Autodesk Inventor part; units mm, degrees
ref_plane "YZ Plane" through (0, 0, 0) normal (1, 0, 0) x (0, 1, 0)
ref_plane "XZ Plane" through (0, 0, 0) normal (0, 1, 0) x (-1, 0, 0)
ref_plane "XY Plane" through (0, 0, 0) normal (0, 0, 1) x (1, 0, 0)
sketch "Эскиз1" plane through (0, 0, 0) normal (0, 0, 1) x (1, 0, 0)
  line L0 (0, 0) -> (18, 0)
  line L1 (18, 0) -> (18, 18)
  line L2 (18, 18) -> (0, 18)
  line L3 (0, 18) -> (0, 0)
  dimension "d0" = 18
  dimension "d1" = 18
extrude "Выдавливание1" add sketch "Эскиз1" along normal blind 2
sketch "Эскиз4" plane through (0, 0, 0) normal (0, 0, -1) x (-1, 0, 0)
  circle A0 centre (-9, 9) radius 4.05
  line L0 (-18, 0) -> (-18, 18)
  line L1 (-18, 9) -> (0, 9)
  line L2 (0, 18) -> (0, 0)
  dimension "d14" = 8.1
extrude "Выдавливание3" cut sketch "Эскиз4" against normal blind 0.3
sketch "Эскиз5" plane through (0, 0, 2) normal (0, 0, 1) x (1, 0, 0)
  circle A0 centre (9, 9) radius 1.75
  circle A1 centre (9, 9) radius 5.714
  line L0 (0, 18) -> (0, 0)
  line L1 (6.1362, 11.8638) -> (0, 18)
  line L2 (18, 0) -> (18, 18)
  line L3 (11.8638, 11.8638) -> (18, 18)
  line L4 (0, 0) -> (18, 0)
  line L5 (0, 0) -> (6.1362, 6.1362)
  line L6 (18, 0) -> (11.8638, 6.1362)
  circle A2 centre (9, 9) radius 4.05
  line L7 (3.0681, 14.9319) -> (4.0681, 14.9319)
  line L8 (3.0681, 3.0681) -> (4.0681, 3.0681)
  line L9 (14.9319, 3.0681) -> (13.9319, 3.0681)
  line L10 (14.9319, 14.9319) -> (13.9319, 14.9319)
  dimension "d24" = 1
hole "Отверстие2" at (4.0681, 14.9319, 2) at (4.0681, 3.0681, 2) at (13.9319, 14.9319, 2) at (13.9319, 3.0681, 2) direction (0, 0, -1) diameter 2.2 depth 5 countersink diameter 4 countersink angle 90
fillet "Сопряжение1" radius 1.05 2 edges at (9, 0, 2) (9, 18, 2)
fillet "Сопряжение1" radius 2.05 2 edges at (18, 9, 2) (0, 9, 2)
sketch "Эскиз6" plane through (9, 9, 0.3) normal (0, 0, -1) x (-1, 0, 0)
  circle A0 centre (0, 0) radius 1.75
  point P0 (9, -9)
  dimension "d27" = 3.5
extrude "Выдавливание4" cut sketch "Эскиз6" against normal through all
properties part number "Крышка поворотного кулака"
Could you check a few things on this model? Use its own coordinates, in mm. A direction names the side the tool comes from. Round coordinates to 2 decimals unless told otherwise and drop trailing zeros. Write each loop counter-clockwise with the first axis right and the second up, starting at its lowest first coordinate (ties: lowest second). Pieces come first, ordered by that corner, then holes. Notation, with made-up numbers: M -14,41.25 L 38,41.25 A20 ccw 38,69.25 Z; hole C -1,35.5 d1. An arc over 180 degrees is marked long. Answer in a Markdown table with one row per item. Add a question column.
Q1. Imagine slicing it at B-B (y = 9). Please give me the cut outline in (x, z), then the cut area to 3 significant figures.
Q2. Will these pins go through, and if not, where does the flat tip stop? pin 1 Ø3 at (x, y) = (4.07, 3.07) entering from -Z; pin 2 Ø3 at (x, y) = (13.93, 14.93) entering from +Z; pin 3 Ø2 at (x, y) = (4.07, 14.93) entering from -Z.
Q3. On a 3-axis mill with a long thin cutter (end or side, diameter ignored), from which of +Z, -Z, +X, -X, +Y, -Y can I reach the whole of each face in a straight line? I mean faces 1 (the cylindrical face through (4.489, 2.052, 0.542)), 2 (the flat face through (7, 8, 0.3)). Say none if no direction works.
Q4. If I drill on line 1 (Y direction, x = 14, z = 0.9); line 2 (Y direction, x = 13.5, z = 1.2); line 3 (X direction, y = 2.5, z = 1.8), over which ranges is the centre line in solid material (lowest first)? Write a range as from..to.
Q5. Imagine slicing it at C-C (z = 1.55). Please give me the cut outline in (x, y), then the cut area to 3 significant figures.
Q6. Imagine slicing it at D-D (x = 7). Please give me the cut outline in (y, z), then the cut area to 3 significant figures.
Q7. Imagine slicing it at A-A (x = 9). Please give me the cut outline in (y, z).
Q8. If we mould it in two halves opening along X, with no side actions, what happens to faces 3 (the flat face through (9, 11, 2)), 4 (the cylindrical face through (0.6, 9.1, 1.4)), 5 (the cylindrical face through (4.489, 13.916, 0.542))? For each: +X half, -X half, draft (parallel to the pull), parting line (faces both ways), or undercut.
Values:
| question | item | result |
|---|---|---|
| 1 | outline | M 0,0 L 4.95,0 L 4.95,0.3 L 7.25,0.3 L 7.25,2 L 2.01,2 A2.05 ccw Z; M 10.75,0.3 L 13.05,0.3 L 13.05,0 L 18,0 A2.05 ccw 15.99,2 L 10.75,2 Z |
| 1 | area | 25.8 mm^2 |
| 2 | pin 1 | z = 0 |
| 2 | pin 2 | z = 1.5 |
| 2 | pin 3 | through |
| 3 | face 1 | +Z, -Z |
| 3 | face 2 | -Z |
| 4 | line 1 | 0..1.97, 4.17..13.83, 16.03..18 |
| 4 | line 2 | 0.03..1.95, 4.19..13.81, 16.05..17.97 |
| 4 | line 3 | 1.17..2.36, 5.78..12.22, 15.64..16.83 |
| 5 | outline | M 0.77,0.19 L 17.23,0.19 L 17.23,17.81 L 0.77,17.81 Z; hole C 4.07,3.07 d3.1; hole C 4.07,14.93 d3.1; hole C 9,9 d3.5; hole C 13.93,3.07 d3.1; hole C 13.93,14.93 d3.1 |
| 5 | area | 250 mm^2 |
| 6 | outline | M 0,0 L 5.48,0 L 5.48,0.3 L 12.52,0.3 L 12.52,0 L 18,0 L 18,0.98 A1.05 ccw 16.98,2 L 1.02,2 A1.05 ccw 0,0.98 Z |
| 6 | area | 33.4 mm^2 |
| 7 | outline | M 0,0 L 4.95,0 L 4.95,0.3 L 7.25,0.3 L 7.25,2 L 1.02,2 A1.05 ccw 0,0.98 Z; M 10.75,0.3 L 13.05,0.3 L 13.05,0 L 18,0 L 18,0.98 A1.05 ccw 16.98,2 L 10.75,2 Z |
| 8 | face 3 | draft |
| 8 | face 4 | -X half |
| 8 | face 5 | undercut |
